Autodesk Inventor part; units mm, degrees
ref_plane "YZ Plane" through (0, 0, 0) normal (1, 0, 0) x (0, 1, 0)
ref_plane "XZ Plane" through (0, 0, 0) normal (0, 1, 0) x (-1, 0, 0)
ref_plane "XY Plane" through (0, 0, 0) normal (0, 0, 1) x (1, 0, 0)
sketch "Sketch1" plane through (0, 0, 0) normal (0, 1, 0) x (-1, 0, 0)
  line L0 (-7.5, -1.5) -> (7.5, -1.5)
  line L1 (7.5, 3.5) -> (7.5, 3.5)
  line L2 (7.5, 1.5) -> (-7.5, 1.5)
  line L3 (-7.5, 3.5) -> (-7.5, 3.5)
  line L4 (-7.5, -1.5) -> (7.5, 1.5) construction
  line L5 (7.5, -1.5) -> (-7.5, 1.5) construction
  circle A0 centre (6, 0) radius 1
  line L6 (-7.5, 1.5) -> (-7.5, -1.5)
  line L7 (7.5, 1.5) -> (7.5, -1.5)
  line L8 (-7.5, -1.5) -> (-4.5, -1.5)
  circle A1 centre (-6, 0) radius 1
  point P0 (0, 0)
  point P1 (-7.5, 0)
  dimension "d0" = 3
  dimension "d1" = 15
  dimension "d3" = 2
  dimension "d6" = 1.5
  dimension "d8" = 1.5
  dimension "d21" = 2
  dimension "d22" = 1.5
  dimension "d23" = 1.5
extrude "Extrusion1" add sketch "Sketch1" along normal blind 5
properties part number "link"
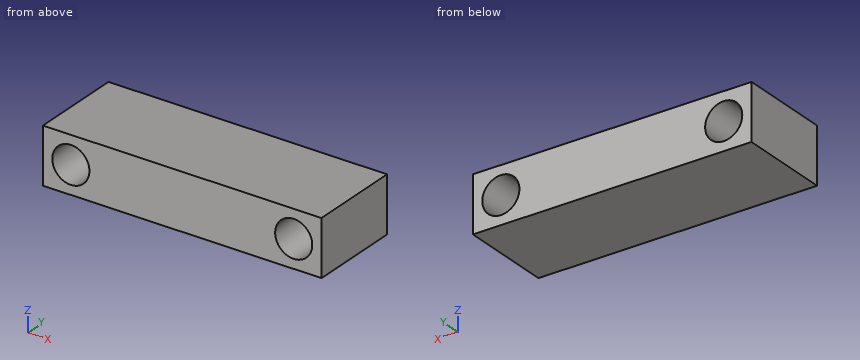
Part model, mm, in its own coordinate system. Coordinates: 2 decimals unless noted, no trailing zeros. Order: outer loops, then holes, each group sorted by start corner. A loop starts at its lowest first (then second) coordinate and runs counter-clockwise, first axis right, second up. Notation, with made-up numbers: (-6.5, -2) - (32.5, -2) arc R34 cw to (32.5, 28) - close; hole circle Ø10 at (41.5, -29). An arc over 180 degrees is marked (long way). Return JSON: item names as keys, results as strings. Group by question number.
Item 1: Cut at C-C (x = 6). List the corners of the cut face in (y, z), plus the area to 3 significant figures.
Item 2: Cut at B-B (y = 1). List the corners of the cut face in (x, z).
Item 3: Cut at A-A (z = 0). List the corners of the cut face in (x, y), plus the area to 3 significant figures.
Item 4: Drill centre lines: probe 1 along X at (y, z) = (4.4, 0.85); probe 2 along Z at (x, y) = (-6, 3.1); probe 3 along X at (y, z) = (4.35, 0.55). Where is each one in solid material? Low to high. Write a range as from..to.
Check values:
{
 "1": {"outline": "(0, -1.5) - (5, -1.5) - (5, -1) - (0, -1) - close; (0, 1) - (5, 1) - (5, 1.5) - (0, 1.5) - close", "area": "5.00 mm2"},
 "2": {"outline": "(-7.5, -1.5) - (7.5, -1.5) - (7.5, 1.5) - (-7.5, 1.5) - close; hole circle Ø2 at (-6, 0); hole circle Ø2 at (6, 0)"},
 "3": {"outline": "(-7.5, 0) - (-7, 0) - (-7, 5) - (-7.5, 5) - close; (-5, 0) - (5, 0) - (5, 5) - (-5, 5) - close; (7, 0) - (7.5, 0) - (7.5, 5) - (7, 5) - close", "area": "55.0 mm2"},
 "4": {"probe 1": "x = -7.5..-6.53, -5.47..5.47, 6.53..7.5", "probe 2": "z = -1.5..-1, 1..1.5", "probe 3": "x = -7.5..-6.84, -5.16..5.16, 6.84..7.5"}
}
